from build123d import *

# Parameters (mm, degrees)
SKETCH1_W           = 20
SKETCH1_H           = 30
BOSS_EXTRUDE1_DEPTH = 3
SKETCH2_W           = 20
SKETCH2_H           = 3
BOSS_EXTRUDE2_DEPTH = 20


with BuildPart() as part:
    # Sketch1 → Boss-Extrude1 (new body)
    with BuildSketch(Plane(origin=(0, 0, 0), x_dir=(0, 0, -1), z_dir=(1, 0, 0))):
        Rectangle(SKETCH1_W, SKETCH1_H)
        with BuildLine():
            Line((-3.5, 10), (-3.5, -10))
            ThreePointArc((-3.5, -10), (-5, -11.5), (-6.5, -10))
            Line((-6.5, -10), (-6.5, 10))
            ThreePointArc((-6.5, 10), (-5, 11.5), (-3.5, 10))
        make_face(mode=Mode.SUBTRACT)
        with BuildLine():
            Line((6.5, 10), (6.5, -10))
            ThreePointArc((6.5, -10), (5, -11.5), (3.5, -10))
            Line((3.5, -10), (3.5, 10))
            ThreePointArc((3.5, 10), (5, 11.5), (6.5, 10))
        make_face(mode=Mode.SUBTRACT)
    extrude(amount=BOSS_EXTRUDE1_DEPTH)

    # Sketch2 → Boss-Extrude2 (add)
    with BuildSketch(Plane(origin=(3, 0, 0), x_dir=(0, 0, -1), z_dir=(1, 0, 0))):
        with Locations((0, 13.5)):
            Rectangle(SKETCH2_W, SKETCH2_H)
    extrude(amount=BOSS_EXTRUDE2_DEPTH)


solid = part.part
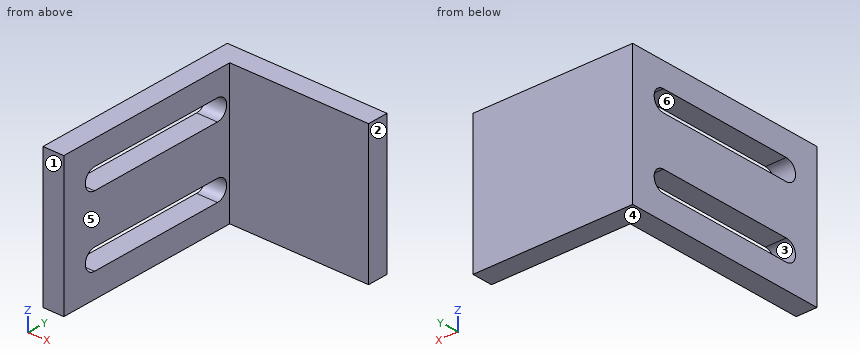
Read the model definition and answer for the solid it produces. Units are mm, in the model's axes. Face numbers are marked on the shaded views. A direction names the side the tool comes from. Give positions to 0.01 mm unless a question says otherwise; leave off trailing zeros. Write each loop counter-clockwise with the first axis right and the second up, starting at its lowest first coordinate (ties: lowest second). Pieces come first, ordered by that corner, then holes. Notation, with made-up numbers: (68.5, 26) - (84.5, 26) arc R19 ccw to (84.5, 62) - close; hole circle Ø4 at (61.5, 15.25). An arc over 180 degrees is marked (long way). Answer in a Markdown table with one row per item. Add a question column.
Item 1: Section C-C, the plane x = 1.75 is taken. Write down the section's boundary in (y, z), and give its area (3 significant figures).
Item 2: Section A-A, the plane y = -2.25 is taken. Write down the section's boundary in (x, z).
Item 3: Section B-B, the plane z = -5 is taken. Write down the section's boundary in (x, y), and give its area (3 significant figures).
Item 4: Find the intervals of material crossed by L1, parallel to Y at x = 10.25, z = 0; L2, parallel to X at y = 2.75, z = 7.5, in increasing order.
Item 5: A tool of negligible diameter and unlimited length cuts with its end or side. For the marked faces 4, 5 and 6, from which of +Z, -Z, +X, -X, +Y, -Y can it reach the whole face along a straight path? Write none if from no direction.
Item 6: Determine the mould class of the marked faces 1, 2 and 3 for opening direction Y: pulls with the +Y half, pulls with the -Y half, needs draft (parallel to the pull), parting line crosses it, or undercut.
Item 7: Section D-D, the plane z = -8 is taken. Write down the section's boundary in (x, y), and give its area (3 significant figures).
Item 8: Flat-ended cylindrical pins translate along their axes: P1, Ø4, axis at y = -2.5, z = 0, coming from the +X side; P2, Ø10, axis at x = 16, z = 5, coming from the -Y side. Find the tip coordinate at first contact, or state that the pin passes through.
Recorded:
| question | item | result |
|---|---|---|
| 1 | outline | (-15, -10) - (15, -10) - (15, 10) - (-15, 10) - close; hole (-10, -6.5) - (10, -6.5) arc R1.5 ccw to (10, -3.5) - (-10, -3.5) arc R1.5 ccw to start; hole (-10, 3.5) - (10, 3.5) arc R1.5 ccw to (10, 6.5) - (-10, 6.5) arc R1.5 ccw to start |
| 1 | area | 466 mm2 |
| 2 | outline | (0, -10) - (3, -10) - (3, -6.5) - (0, -6.5) - close; (0, -3.5) - (3, -3.5) - (3, 3.5) - (0, 3.5) - close; (0, 6.5) - (3, 6.5) - (3, 10) - (0, 10) - close |
| 3 | outline | (0, -15) - (3, -15) - (3, -11.5) - (0, -11.5) - close; (0, 11.5) - (3, 11.5) - (3, 12) - (23, 12) - (23, 15) - (0, 15) - close |
| 3 | area | 81.0 mm2 |
| 4 | L1 | y = 12 to 15 |
| 4 | L2 | x = 0 to 3 |
| 5 | face 4 | -Z, +X, -X, +Y, -Y |
| 5 | face 5 | +Z, -Z, +X, -Y |
| 5 | face 6 | +X, -X |
| 6 | face 1 | pulls with the -Y half |
| 6 | face 2 | needs draft |
| 6 | face 3 | undercut |
| 7 | outline | (0, -15) - (3, -15) - (3, 12) - (23, 12) - (23, 15) - (0, 15) - close |
| 7 | area | 150 mm2 |
| 8 | P1 | stops at x = 3 |
| 8 | P2 | stops at y = 12 |
